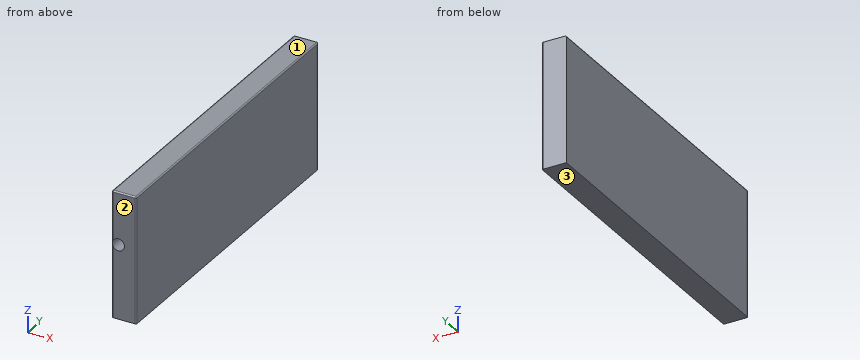
from build123d import *

# Parameters (mm, degrees)
F0_W         = 97.7746620774
F0_H         = 1270
F1_DEPTH     = 508
F2_R         = 24.2123900656
F3_DEPTH     = 762
F4_T1_DEPTH  = 87.6146620774
F4_T3_DEPTH  = 1277.62
F4_T5_DEPTH  = 515.62
F4_T7_DEPTH  = 533.4
F4_S11_W     = 5.08
F4_S11_H     = 5.08
F4_T12_DEPTH = 5.08
F4_S17_W     = 5.08
F4_S17_H     = 5.08
F4_T18_DEPTH = 5.08


# Not quite as in the source:
# - a fillet or chamfer that OpenCascade refuses, or shapes differently, is made with other operations: its cross-section is extruded or revolved along the edge and cut away or added


with BuildPart() as f1:
    # F0 (on Top) → F1 (new body)
    with BuildSketch(Plane.XY):
        with Locations((-1.3020187616, 606.1489956826)):
            Rectangle(F0_W, F0_H)
    extrude(amount=F1_DEPTH)

    # F2 (on face) → F3 (cut)
    with BuildSketch(Plane.XZ.offset(28.8510043174)):
        with Locations((-24.6240980923, 297.7288961411)):
            Circle(F2_R)
    extrude(amount=-F3_DEPTH, mode=Mode.SUBTRACT)

    # F4: fillet of radius 5.08 on 6 edges, made by hand

    # F4_s2 → F4_t1 (cut)
    with BuildSketch(Plane.YZ.offset(-45.1093498003)):
        with BuildLine():
            ThreePointArc((-23.7710043174, 508), (-27.3631067658, 506.5121024484), (-28.8510043174, 502.92))
            Line((-28.8510043174, 502.92), (-28.8510043174, 508))
            Line((-28.8510043174, 508), (-23.7710043174, 508))
        make_face()
    extrude(amount=F4_T1_DEPTH, mode=Mode.SUBTRACT)

    # F4_s4 → F4_t3 (cut)
    with BuildSketch(Plane.XZ.offset(-1253.8489956826)):
        with BuildLine():
            ThreePointArc((47.5853122771, 502.92), (46.0974147255, 506.5121024484), (42.5053122771, 508))
            Line((42.5053122771, 508), (47.5853122771, 508))
            Line((47.5853122771, 508), (47.5853122771, 502.92))
        make_face()
        with BuildLine():
            ThreePointArc((-50.1893498003, 502.92), (-48.7014522488, 506.5121024484), (-45.1093498003, 508))
            Line((-45.1093498003, 508), (-50.1893498003, 508))
            Line((-50.1893498003, 508), (-50.1893498003, 502.92))
        make_face()
    extrude(amount=F4_T3_DEPTH, mode=Mode.SUBTRACT)

    # F4_s6 → F4_t5 (cut)
    with BuildSketch(Plane.XY.offset(-12.7)):
        with BuildLine():
            ThreePointArc((47.5853122771, -23.7710043174), (46.0974147255, -27.3631067658), (42.5053122771, -28.8510043174))
            Line((42.5053122771, -28.8510043174), (47.5853122771, -28.8510043174))
            Line((47.5853122771, -28.8510043174), (47.5853122771, -23.7710043174))
        make_face()
        with BuildLine():
            ThreePointArc((-50.1893498003, -23.7710043174), (-48.7014522488, -27.3631067658), (-45.1093498003, -28.8510043174))
            Line((-45.1093498003, -28.8510043174), (-50.1893498003, -28.8510043174))
            Line((-50.1893498003, -28.8510043174), (-50.1893498003, -23.7710043174))
        make_face()
    extrude(amount=F4_T5_DEPTH, mode=Mode.SUBTRACT)

    # F4_s8 → F4_t7 (cut)
    with BuildSketch(Plane.XY.offset(-12.7)):
        with BuildLine():
            ThreePointArc((42.5053122771, 1241.1489956826), (46.0974147255, 1239.661098131), (47.5853122771, 1236.0689956826))
            Line((47.5853122771, 1236.0689956826), (47.5853122771, 1241.1489956826))
            Line((47.5853122771, 1241.1489956826), (42.5053122771, 1241.1489956826))
        make_face()
    extrude(amount=F4_T7_DEPTH, mode=Mode.SUBTRACT)


with BuildPart() as f4_tool10:
    # F4_s11 → F4_t12 (new body)
    with BuildSketch(Plane.YZ.offset(-45.1093498003)):
        with Locations((-26.3110043174, 505.46)):
            Rectangle(F4_S11_W, F4_S11_H)
    extrude(amount=-F4_T12_DEPTH)

    # F4_s13 → F4_t14 (revolve, cut)
    with BuildSketch(Plane(origin=(-45.1093498003, -23.7710043174, 502.92), x_dir=(0, 0.7071067812, -0.7071067812), z_dir=(0, 0.7071067812, 0.7071067812))):
        with BuildLine():
            ThreePointArc((0, -5.08), (5.08, 0), (0, 5.08))
            Line((0, 5.08), (0, -5.08))
        make_face()
    revolve(axis=Axis((-45.1093498003, -23.7710043174, 502.92), (-1, 0, 0)), mode=Mode.SUBTRACT)


with BuildPart() as f1_1:
    add(f1.part)

    # F4_t9: cut F4_tool10
    add(f4_tool10.part, mode=Mode.SUBTRACT)


with BuildPart() as f4_tool16:
    # F4_s17 → F4_t18 (new body)
    with BuildSketch(Plane.YZ.offset(42.5053122771)):
        with Locations((-26.3110043174, 505.46)):
            Rectangle(F4_S17_W, F4_S17_H)
    extrude(amount=F4_T18_DEPTH)

    # F4_s19 → F4_t20 (revolve, cut)
    with BuildSketch(Plane(origin=(42.5053122771, -23.7710043174, 502.92), x_dir=(0, 0.7071067812, -0.7071067812), z_dir=(0, -0.7071067812, -0.7071067812))):
        with BuildLine():
            ThreePointArc((0, -5.08), (5.08, 0), (0, 5.08))
            Line((0, 5.08), (0, -5.08))
        make_face()
    revolve(axis=Axis((42.5053122771, -23.7710043174, 502.92), (1, 0, 0)), mode=Mode.SUBTRACT)


with BuildPart() as f1_2:
    add(f1_1.part)

    # F4_t15: cut F4_tool16
    add(f4_tool16.part, mode=Mode.SUBTRACT)


solid = f1_2.part
The model under review builds one solid part; all positions refer to its coordinate system, in mm. Face numbers are marked on the shaded views. Coordinates: 2 decimals unless noted, no trailing zeros. Loops run counter-clockwise (first coordinate to the right, second up) from the corner with the lowest first, then second, coordinate; pieces in that order, holes last.
(1) Consider section B-B, the plane x = -33. Give the boundary of the cut face in (y, z), plus the area to 3 significant figures.
Determined:
outline: (-28.85, 0) - (1241.15, 0) - (1241.15, 508) - (-23.77, 508) arc R5.08 ccw to (-28.85, 502.92) - (-28.85, 320.45) - (733.15, 320.45) - (733.15, 275.01) - (-28.85, 275.01) - close
area: 611,000 mm2
(2) Draft analysis for pull direction Z (two halves, no side actions). For the marked faces 1, 2 and 3, state which applies: +Z half, -Z half, draft (parallel to the pull), parting line (faces both ways), or undercut.
Determined:
face 1: +Z half
face 2: draft
face 3: -Z half
(3) Wall thickness on L1, parallel to Z at x = -21.5, y = 150.5; L2, parallel to Y at x = -34.5, z = 305.5; L3, parallel to Z at x = -33, y = 96: over which ranges is each line inside the solid? List them lowest first.
Determined:
L1: z = 0 to 273.72, 321.74 to 508
L2: y = 733.15 to 1241.15
L3: z = 0 to 275.01, 320.45 to 508
(4) Consider section A-A, the plane y = 163.5. Give the boundary of the cut face in (x, z).
Determined:
outline: (-50.19, 0) - (47.59, 0) - (47.59, 502.92) arc R5.08 ccw to (42.51, 508) - (-45.11, 508) arc R5.08 ccw to (-50.19, 502.92) - close; hole circle Ø48.42 at (-24.62, 297.73)
